Verification items for the finished model (mm, model axes). A direction names the side the tool comes from. Round coordinates to 2 decimals unless told otherwise and drop trailing zeros. Write each loop counter-clockwise with the first axis right and the second up, starting at its lowest first coordinate (ties: lowest second). Pieces come first, ordered by that corner, then holes. Notation, with made-up numbers: M 17.5,71.25 L 61.5,71.25 A12 cw 61.5,93.25 Z; hole C 37,59 d10. An arc over 180 degrees is marked long. One line per question, with ' | ' between items. Start each with the question number.
Q1. Thickness scan on line 1 along X through (y, z) = (36, 36); line 2 along Y through (x, z) = (-185, 3); line 3 along Z through (x, y) = (-48.5, -46). Record the ranges inside material, lowest first. Write a range as from..to.
Q2. Tool access check on faces 4 (the face through (-167, -22.5, 0)), 5 (the face through (-130, 1, 1)), 6 (the face through (140.14, 20.765, -39.923)), 7 (the face through (-172, 0, -7.25)). Record the directions out of +Z, -Z, +X, -X, +Y, -Y that give a thin tool (end or side, any length) a straight path to the whole face; none if there is none.
Q3. Cross-section at D-D (y = -28). Record the boundary of the cut face in (x, z), then the cut area to 3 significant figures.
Q4. Cross-section at C-C (x = -122). Record the boundary of the cut face in (y, z), then the cut area to 3 significant figures.
Q5. Release check for a two-part mould opening along Z. For faces 1 (the face through (1.82, -11.923, -53.692)), 2 (the face through (-168, 22.5, 0)), 3 (the face through (-172, 0, 7.25)) record: released by +Z, released by -Z, zero draft, split by the parting line, or undercut.
Q6. Gauge pin test, flat ends, axial feed: pin 1 (2 mm diameter, centred on x = -42, z = 27.5, fed in from +Y); pin 2 (3 mm diameter, centred on y = -8.5, z = -48, fed in from -X); pin 3 (12 mm diameter, centred on x = -82, y = -45, fed in from +Z). Record the tip position at first contact, or that the pin passes through.
Q7. Cross-section at A-A (y = 0). Record the boundary of the cut face in (x, z), then the cut area to 3 significant figures.
Q8. Cross-section at B-B (z = 0). Record the boundary of the cut face in (x, y), then the cut area to 3 significant figures.
from build123d import *

# Parameters (mm, degrees)
SKETCH3_R                = 10
BOSS_EXTRUDE1_DEPTH      = 7.25
BOSS_EXTRUDE1_DEPTH_BACK = 7.25


with BuildPart() as part:
    # Sketch1 → Revolve1 (revolve)
    with BuildSketch(Plane.XY):
        Polygon((150, 45), (150, 60), (-150, 60), (-150, 0), (-130, 0), (-130, 55), (130, 55), (130, 45), align=None)
    revolve(axis=Axis((-150, 0, 0), (1, 0, 0)))

    # Sketch3 → Boss-Extrude1 (add, two sides)
    with BuildSketch(Plane.XY) as boss_extrude1_sk:
        with BuildLine():
            Line((-150, 22.5), (-150, -22.5))
            Line((-150, -22.5), (-185, -22.5))
            ThreePointArc((-185, -22.5), (-207.5, 0), (-185, 22.5))
            Line((-185, 22.5), (-150, 22.5))
        make_face()
        with Locations((-185, 0)):
            Circle(SKETCH3_R, mode=Mode.SUBTRACT)
    extrude(amount=BOSS_EXTRUDE1_DEPTH)
    extrude(boss_extrude1_sk.sketch, amount=-BOSS_EXTRUDE1_DEPTH_BACK)


solid = part.part
Determined:
1) line 1: x = -150..-130, 130..150 | line 2: y = -22.5..-10, 10..22.5 | line 3: z = -38.52..-30.15, 30.15..38.52
2) face 4: +Z, -Z, -X, -Y | face 5: none | face 6: +X | face 7: -Z, -X, +Y, -Y
3) outline: M -150,-53.07 L 150,-53.07 L 150,-35.23 L 130,-35.23 L 130,-47.34 L -130,-47.34 L -130,47.34 L 130,47.34 L 130,35.23 L 150,35.23 L 150,53.07 L -150,53.07 Z | area: 5,810 mm²
4) outline: C 0,0 d120; hole C 0,0 d110 | area: 1,810 mm²
5) face 1: undercut | face 2: zero draft | face 3: released by +Z
6) pin 1: stops at y = 53.83 | pin 2: stops at x = -150 | pin 3: stops at z = 45.6
7) outline: M -207.5,-7.25 L -195,-7.25 L -195,7.25 L -207.5,7.25 Z; M -175,-7.25 L -150,-7.25 L -150,-60 L 150,-60 L 150,-45 L 130,-45 L 130,-55 L -130,-55 L -130,55 L 130,55 L 130,45 L 150,45 L 150,60 L -150,60 L -150,7.25 L -175,7.25 Z | area: 6,140 mm²
8) outline: M -185,-22.5 L -150,-22.5 L -150,-60 L 150,-60 L 150,-45 L 130,-45 L 130,-55 L -130,-55 L -130,55 L 130,55 L 130,45 L 150,45 L 150,60 L -150,60 L -150,22.5 L -185,22.5 A22.5 ccw Z; hole C -185,0 d20 | area: 7,660 mm²
